Geometry check sheet. Reference: the model listing, model coordinates, mm. A direction names the side the tool comes from. Give positions to 0.01 mm unless a question says otherwise; leave off trailing zeros. Write each loop counter-clockwise with the first axis right and the second up, starting at its lowest first coordinate (ties: lowest second). Pieces come first, ordered by that corner, then holes. Notation, with made-up numbers: (32, -18) -> (42, -18) arc R13 cw to (42, -3) -> close; hole circle Ø11 at (39, 70.5). An arc over 180 degrees is marked (long way). One line per item, written item: value.
Autodesk Fusion 360 part; units mm, degrees
sketch "Sketch3" plane through (0, 0, 0) normal (0, 0, 1) x (1, 0, 0)
  circle A0 centre (0, 0) radius 5.08
  dimension "d5" = 10.16
extrude "Extrude2" add sketch "Sketch3" along normal blind 7.62
sketch "Sketch4" plane through (0, 0, 7.62) normal (0, 0, 1) x (-1, 0, 0)
  circle A0 centre (0, 0) radius 5.08
  circle A1 centre (0, 0) radius 10.795
  dimension "d8" = 21.59
extrude "Extrude3" add sketch "Sketch4" along normal blind 86.36 contours A0 | A1
sketch "Sketch7" plane through (0, 0, 93.98) normal (0, 0, 1) x (-1, 0, 0)
  circle A0 centre (0, 0) radius 10.795
  circle A1 centre (0, 0) radius 12.7
  circle A2 centre (-12.7, -0.0001) radius 4.5016
  circle A3 centre (12.6996, -0.1003) radius 4.5018
  line L0 (15.5784, -3.5613) -> (8.1213, -9.7639)
  line L1 (-8.1983, -9.6993) -> (-15.606, -3.4381)
  line L2 (-15.606, 3.4379) -> (-8.1984, 9.6993)
  line L3 (8.2745, 9.6344) -> (15.6327, 3.3149)
  circle A4 centre (0, 0) radius 12.7
  dimension "d14" = 25.4
extrude "Extrude4" add sketch "Sketch7" along normal blind 2.54
sketch "Sketch8" plane through (0, 0, 96.52) normal (0, 0, 1) x (-1, 0, 0)
  arc A0 (-15.606, 3.4379) -> (-15.606, -3.4381) centre (-12.7, -0.0001) ccw
  line L0 (-15.606, -3.4381) -> (-8.1983, -9.6993)
  arc A1 (-8.1983, -9.6993) -> (8.1213, -9.7639) centre (0, 0) ccw
  line L1 (8.1213, -9.7639) -> (15.5784, -3.5613)
  arc A2 (15.5784, -3.5613) -> (15.6327, 3.3149) centre (12.6996, -0.1003) ccw
  line L2 (15.6327, 3.3149) -> (8.2745, 9.6344)
  arc A3 (8.2745, 9.6344) -> (-8.1984, 9.6993) centre (0, 0) ccw
  line L3 (-8.1984, 9.6993) -> (-15.606, 3.4379)
  circle A4 centre (0, 0) radius 9.779
  dimension "d15" = 19.558
extrude "Extrude5" cut sketch "Sketch8" against normal blind 86.36 contours A4
1) Mould release check, pull along Y, two halves, no side actions. Record for faces 1 (the flat face through (0, 0, 10.16)), 2 (the flat face through (8, -8, 93.98)), 3 (the flat face through (-11.9, 6.62, 95.23)), 4 (the flat face through (-11.9, -6.52, 95.23)): released by +Y, released by -Y, zero draft, split by the parting line, or undercut.
Verdict:
face 1: undercut
face 2: zero draft
face 3: released by +Y
face 4: released by -Y
2) Sectioned sample at B-B on z = 86.5. Record the cut outline in (x, y) (3 decimals), plus the area to 3 significant figures.
Verdict:
outline: circle Ø21.59 at (0, 0); hole circle Ø19.558 at (0, 0)
area: 65.7 mm^2
3) Tool access check on faces 5 (the flat face through (-5, 2, 7.62)), 6 (the cylindrical face through (2.12, 9.546, 53.945)), 7 (the flat face through (11.954, -6.525, 95.232)). Record the directions out of +Z, -Z, +X, -X, +Y, -Y that give a thin tool (end or side, any length) a straight path to the whole face; none if there is none.
Verdict:
face 5: -Z
face 6: +Z
face 7: +Z, -Z, +X, -Y
4) Sectioned sample at C-C on y = -2. Record the cut outline in (x, z), plus the area to 3 significant figures.
Verdict:
outline: (-16.68, 93.98) -> (-10.61, 93.98) -> (-10.61, 7.62) -> (-4.67, 7.62) -> (-4.67, 0) -> (4.67, 0) -> (4.67, 7.62) -> (10.61, 7.62) -> (10.61, 93.98) -> (16.73, 93.98) -> (16.73, 96.52) -> (9.57, 96.52) -> (9.57, 10.16) -> (-9.57, 10.16) -> (-9.57, 96.52) -> (-16.68, 96.52) -> close
area: 335 mm^2
5) Scan lines: probe 1 along X at (y, z) = (0, 69) (3 decimals); probe 2 along Z at (x, y) = (-15, -3.25). Record each from-to range of solid material in increasing order.
Verdict:
probe 1: -10.795 to -9.779, 9.779 to 10.795
probe 2: 93.98 to 96.52
6) Sectioned sample at A-A on x = 0. Record the cut outline in (y, z) (3 decimals), plus the area to 3 significant figures.
Verdict:
outline: (-12.7, 93.98) -> (-10.795, 93.98) -> (-10.795, 7.62) -> (-5.08, 7.62) -> (-5.08, 0) -> (5.08, 0) -> (5.08, 7.62) -> (10.795, 7.62) -> (10.795, 93.98) -> (12.7, 93.98) -> (12.7, 96.52) -> (9.779, 96.52) -> (9.779, 10.16) -> (-9.779, 10.16) -> (-9.779, 96.52) -> (-12.7, 96.52) -> close
area: 317 mm^2
7) Sectioned sample at D-D on x = 12. Record the cut outline in (y, z), plus the area to 3 significant figures.
Verdict:
outline: (-6.49, 93.98) -> (6.49, 93.98) -> (6.49, 96.52) -> (-6.49, 96.52) -> close
area: 32.9 mm^2
8) Depth check by flat-ended pin: pin 1 Ø8 at (y, z) = (1, 15) entering from +X (3 decimals); pin 2 Ø10 at (x, z) = (3.5, 68) entering from -Y (3 decimals); pin 3 Ø5 at (y, z) = (-7.5, 31.5) entering from +X. Enter the tip coordinate at first touch or a pass-through.
Verdict:
pin 1: x = 10.795
pin 2: y = -10.795
pin 3: x = 9.57
